from build123d import *

# Parameters (mm, degrees)
F1_DEPTH = 20
F3_DEPTH = 25
F4_DEPTH = 25


with BuildPart() as f1:
    # F0 (on Top) → F1 (new body)
    with BuildSketch(Plane.XY):
        with BuildLine():
            ThreePointArc((-2.5275626504, 0), (-2.6688577349, 0.0041097327), (-2.8101528193, 0))
            Line((-2.8101528193, 0), (-2.5275626504, 0))
        make_face()
        with BuildLine():
            ThreePointArc((-0.2378978583, -2.4268501438), (-0.900659697, -0.7586050718), (-2.5275626504, 0))
            Line((-2.5275626504, 0), (-2.5275626504, -0.7201090608))
            ThreePointArc((-2.5275626504, -0.7201090608), (-1.4089155682, -1.2669039546), (-0.9562779775, -2.4268501438))
            ThreePointArc((-0.9562779775, -2.4268501438), (-2.3780599484, -4.1145604485), (-4.2826819718, -3))
            Line((-4.2826819718, -3), (-5.0312855462, -3))
            ThreePointArc((-5.0312855462, -3), (-2.3802414664, -4.8406161994), (-0.2378978583, -2.4268501438))
        make_face()
        with BuildLine():
            Line((-2.5275626504, 0), (-2.8101528193, 0))
            ThreePointArc((-2.8101528193, 0), (-4.6226123471, -0.9803340406), (-5.0312855462, -3))
            Line((-5.0312855462, -3), (-4.2826819718, -3))
            ThreePointArc((-4.2826819718, -3), (-4.0258990754, -1.3821644373), (-2.5275626504, -0.7201090608))
            Line((-2.5275626504, -0.7201090608), (-2.5275626504, 0))
        make_face()
        with BuildLine():
            Line((-2.8101528193, 0), (-27.5275626504, 0))
            Line((-27.5275626504, 0), (-27.5275626504, -3))
            Line((-27.5275626504, -3), (-5.0312855462, -3))
            ThreePointArc((-5.0312855462, -3), (-4.6226123471, -0.9803340406), (-2.8101528193, 0))
        make_face()
    extrude(amount=F1_DEPTH)

    # F2 (on face) → F3 (cut)
    with BuildSketch(Plane(origin=(0, 0, 0), x_dir=(-1, 0, 0), z_dir=(0, 1, 0))):
        with BuildLine():
            Line((22.7848533541, 5), (22.7848533541, 2.5))
            ThreePointArc((22.7848533541, 2.5), (24.5526203071, 3.232233047), (25.2848533541, 5))
            ThreePointArc((25.2848533541, 5), (24.5526203071, 6.767766953), (22.7848533541, 7.5))
            Line((22.7848533541, 7.5), (22.7848533541, 5))
        make_face()
        with BuildLine():
            Line((22.7848533541, 15), (22.7848533541, 12.5))
            ThreePointArc((22.7848533541, 12.5), (24.5526203071, 13.232233047), (25.2848533541, 15))
            ThreePointArc((25.2848533541, 15), (24.5526203071, 16.767766953), (22.7848533541, 17.5))
            Line((22.7848533541, 17.5), (22.7848533541, 15))
        make_face()
        with BuildLine():
            ThreePointArc((22.7848533541, 17.5), (20.2848533541, 15), (22.7848533541, 12.5))
            Line((22.7848533541, 12.5), (22.7848533541, 15))
            Line((22.7848533541, 15), (22.7848533541, 17.5))
        make_face()
    extrude(amount=-F3_DEPTH, mode=Mode.SUBTRACT)

    # F2 (on face) → F4 (cut)
    with BuildSketch(Plane(origin=(0, 0, 0), x_dir=(-1, 0, 0), z_dir=(0, 1, 0))):
        with BuildLine():
            ThreePointArc((22.7848533541, 7.5), (20.2848533541, 5), (22.7848533541, 2.5))
            Line((22.7848533541, 2.5), (22.7848533541, 5))
            Line((22.7848533541, 5), (22.7848533541, 7.5))
        make_face()
    extrude(amount=-F4_DEPTH, mode=Mode.SUBTRACT)


solid = f1.part
Can you work these out from the model? Positions are in its coordinate system, mm. A direction names the side the tool comes from. Round coordinates to 2 decimals unless told otherwise and drop trailing zeros. Loops run counter-clockwise (first coordinate to the right, second up) from the corner with the lowest first, then second, coordinate; pieces in that order, holes last. Notation, with made-up numbers: (-35.75, 9) - (1.25, 9) arc R28 ccw to (1.25, 40) - close; hole circle Ø5 at (81.5, 73.5). An arc over 180 degrees is marked (long way). Use CSV: the item, a comma, the result in double quotes. Start each with the question number.
1) If we section it at D-D on z = 8: Write out the boundary of the cut face in (x, y), plus the area to 3 significant figures.
2) Please list where these lines run through material, in increasing order: probe 1 along X at (y, z) = (-2.85, 3.25) (1 decimal); probe 2 along Y at (x, z) = (-17.25, 19); probe 3 along Y at (x, z) = (-2, 3). Write a range as [from, to].
3) If we section it at B-B on y = -1.95: Write out the boundary of the cut face in (x, z).
4) For pin 1 Ø10 at (x, z) = (-16, 13) entering from +Y; pin 2 Ø2 at (y, z) = (-1, 15.5) entering from +X, each with a flat end and sliding along its axis, tell me the tip position at first contact or that it passes through.
5) If we section it at A-A on z = 3.5: Write out the boundary of the cut face in (x, y).
6) For faces 1 (the flat face through (-14, -2, 20)), 2 (the flat face through (-16, -3, 10)), which set-ups out of +Z, -Z, +X, -X, +Y, -Y let a thin tool reach every point of the face, with its end or its side?
7) If we section it at C-C on x = -24.25: Write out the boundary of the cut face in (y, z).
Geometry results:
1,outline,"(-27.53, -3) - (-5.03, -3) arc R2.43 ccw (long way) to (-2.81, 0) - (-27.53, 0) - close; hole circle Ø3.43 at (-2.67, -2.43)"
1,area,"77.9 mm2"
2,probe 1,"x = [-27.5, -24.6], [-21, -4.3], [-1, -0.3]"
2,probe 2,"y = [-3, 0]"
2,probe 3,"y = [-4.76, -4], [-0.85, -0.09]"
3,outline,"(-27.53, 0) - (-4.31, 0) - (-4.31, 20) - (-27.53, 20) - close; (-1.02, 0) - (-0.29, 0) - (-0.29, 20) - (-1.02, 20) - close; hole circle Ø5 at (-22.78, 5); hole circle Ø5 at (-22.78, 15)"
4,pin 1,"stops at y = 0"
4,pin 2,"stops at x = -0.28"
5,outline,"(-27.53, -3) - (-24.78, -3) - (-24.78, 0) - (-27.53, 0) - close; (-20.78, -3) - (-5.03, -3) arc R2.43 ccw (long way) to (-2.81, 0) - (-20.78, 0) - close; hole circle Ø3.43 at (-2.67, -2.43)"
6,face 1,"+Z, +X, -X, +Y, -Y"
6,face 2,"+Z, -Z, -X, -Y"
7,outline,"(-3, 0) - (0, 0) - (0, 2.97) - (-3, 2.97) - close; (-3, 7.03) - (0, 7.03) - (0, 12.97) - (-3, 12.97) - close; (-3, 17.03) - (0, 17.03) - (0, 20) - (-3, 20) - close"
